from build123d import *

# Parameters (mm, degrees)
PAD_DEPTH       = 3.95
SKETCH001_W     = 110
SKETCH001_H     = 39.3
PAD001_DEPTH    = 50
SKETCH002_W     = 34.4
SKETCH002_H     = 46
POCKET_DEPTH    = 107
SKETCH003_W     = 46.5
SKETCH003_H     = 35
POCKET001_DEPTH = 40
CHAMFER_SIZE    = 2.5
CHAMFER001_SIZE = 5
FILLET_R        = 2.5
FILLET001_R     = 1
FILLET002_R     = 5
FILLET003_R     = 1


with BuildPart() as part:
    # Sketch → Pad (new body)
    with BuildSketch(Plane.XY):
        Polygon((7.25, 19.75), (45, 19.75), (45, -19.75), (24.75, -19.75), (24.75, -45.2), (63.35, -45.2), (63.35, -109.5), (-46.65, -109.5), (-46.65, -70.2), (-6.65, -70.2), (-6.65, -45.2), (7.25, -45.2), align=None)
    extrude(amount=PAD_DEPTH)

    # Sketch001 (on Face14 of Pad) → Pad001 (join)
    with BuildSketch(Plane.XY.offset(3.95)):
        with Locations((8.35, -89.85)):
            Rectangle(SKETCH001_W, SKETCH001_H)
    extrude(amount=PAD001_DEPTH)

    # Sketch002 (on Face15 of Pad001) → Pocket (cut)
    with BuildSketch(Plane.YZ.offset(63.35)):
        with Locations((-89.8, 28)):
            Rectangle(SKETCH002_W, SKETCH002_H)
    extrude(amount=-POCKET_DEPTH, mode=Mode.SUBTRACT)

    # Sketch003 (on Face1 of Pocket) → Pocket001 (cut)
    with BuildSketch(Plane.XY.offset(53.95)):
        with Locations((-17.9, -87.7)):
            Rectangle(SKETCH003_W, SKETCH003_H)
        with Locations((33.6, -87.7)):
            Rectangle(SKETCH003_W, SKETCH003_H)
    extrude(amount=-POCKET001_DEPTH, mode=Mode.SUBTRACT)

    # Chamfer
    chamfer_edges = [part.edges().sort_by_distance(p)[0] for p in [
        (7.25, 19.75, 1.975),
    ]]
    chamfer(chamfer_edges, length=CHAMFER_SIZE)

    # Chamfer001
    chamfer001_edges = [part.edges().sort_by_distance(p)[0] for p in [
        (63.35, -45.2, 1.975),
    ]]
    chamfer(chamfer001_edges, length=CHAMFER001_SIZE)

    # Fillet
    fillet_edges = [part.edges().sort_by_distance(p)[0] for p in [
        (-6.65, -45.2, 1.975),
        (-6.65, -70.2, 1.975),
    ]]
    fillet(fillet_edges, radius=FILLET_R)

    # Fillet001
    fillet001_edges = [part.edges().sort_by_distance(p)[0] for p in [
        (9.85, -107, 51),
        (9.85, -107, 5),
        (9.85, -72.6, 5),
        (60.1, -72.6, 51),
        (7.85, -72.6, 51),
        (-42.4, -72.6, 51),
    ]]
    fillet(fillet001_edges, radius=FILLET001_R)

    # Fillet002
    fillet002_edges = [part.edges().sort_by_distance(p)[0] for p in [
        (-41.15, -105.2, 52.475),
        (5.35, -105.2, 52.475),
        (10.35, -105.2, 52.475),
        (56.85, -105.2, 52.475),
        (-41.15, -71.4, 13.95),
        (5.35, -71.4, 13.95),
        (10.35, -71.4, 13.95),
        (56.85, -71.4, 13.95),
        (-43.9, -70.2, 53.95),
        (7.85, -70.2, 53.95),
        (60.1, -70.2, 53.95),
    ]]
    fillet(fillet002_edges, radius=FILLET002_R)

    # Fillet003
    fillet003_edges = [part.edges().sort_by_distance(p)[0] for p in [
        (8.35, -109.5, 53.95),
        (-46.65, -109.5, 26.975),
        (63.35, -109.5, 26.975),
        (-46.65, -92.35, 53.95),
        (-46.65, -71.664466, 52.485534),
        (-46.65, -70.2, 24.475),
        (63.35, -70.2, 26.45),
        (63.35, -71.664466, 52.485534),
        (63.35, -92.35, 53.95),
        (8.35, -109.5, 0),
    ]]
    fillet(fillet003_edges, radius=FILLET003_R)


solid = part.part
Geometry check sheet. Reference: the model listing, model coordinates, mm. A direction names the side the tool comes from. Round coordinates to 2 decimals unless told otherwise and drop trailing zeros. Order: outer loops, then holes, each group sorted by start corner. A loop starts at its lowest first (then second) coordinate and runs counter-clockwise, first axis right, second up. Notation, with made-up numbers: M 52,-33 L 60,-33 A8 cw 60,-27 Z; hole C -8.5,61 d3. An arc over 180 degrees is marked long. Answer in a Markdown table with one row per item. Add a question column.
Item 1: Sectioned sample at D-D, the plane x = -12. Enter the section's corners in (y, z), plus the area to 3 significant figures.
Item 2: Sectioned sample at A-A, the plane y = -95.5. Enter the section's corners in (x, z), plus the area to 3 significant figures.
Item 3: Sectioned sample at C-C, the plane x = 28. Enter the section's corners in (y, z).
Item 4: Draft check along X on faces 5 (the face through (3.85, -103.77, 52.45)), 6 (the face through (20, -35, 3.95)), 7 (the face through (-6.65, -58, 2)). Enter one of: released by +X, released by -X, zero draft, split by the parting line, or undercut.
Item 5: Set-up check for faces 1 (the face through (35, -19.75, 2)), 2 (the face through (-41.15, -72, 44)), 3 (the face through (-43.65, -90, 28)), 4 (the face through (9, -58, 0)): record each of +Z, -Z, +X, -X, +Y, -Y from which the full face is reachable in a straight line by a thin tool's end or side.
Item 6: Depth check by flat-ended pin: pin 1 Ø1.2 at (y, z) = (-37.5, 2) entering from +X; pin 2 Ø4.5 at (x, z) = (3.5, 2.5) entering from +Y; pin 3 Ø3 at (y, z) = (-1, 2.5) entering from -X. Enter the tip coordinate at first touch or a pass-through.
Item 7: Material ranges on L1, parallel to Y at x = 47, z = 10; L2, parallel to Y at x = 32, z = 3; L3, parallel to Z at x = -41, y = -78, recorded low to high. Write a range as [from, to].
Item 8: Sectioned sample at B-B, the plane z = 21. Enter the section's corners in (x, y).
Filled in:
| question | item | result |
|---|---|---|
| 1 | outline | M -109.5,1 A1 ccw -108.5,0 L -70.2,0 L -70.2,13.95 L -72.6,13.95 L -72.6,6 A1 cw -73.6,5 L -106,5 A1 cw -107,6 L -107,50 A1 cw -106,51 L -105.2,51 L -105.2,53.95 L -108.5,53.95 A1 ccw -109.5,52.95 Z |
| 1 | area | 346 mm² |
| 2 | outline | M -46.65,0 L 63.35,0 L 63.35,5 L -43.65,5 L -43.65,51 L -41.15,51 L -41.15,53.95 L -45.65,53.95 A1 ccw -46.65,52.95 Z; M 5.35,51 L 10.35,51 L 10.35,53.95 L 5.35,53.95 Z; M 56.85,51 L 63.35,51 L 63.35,52.95 A1 ccw 62.35,53.95 L 56.85,53.95 Z |
| 2 | area | 738 mm² |
| 3 | outline | M -109.5,1 A1 ccw -108.5,0 L -45.2,0 L -45.2,3.95 L -70.2,3.95 L -70.2,13.95 L -72.6,13.95 L -72.6,6 A1 cw -73.6,5 L -106,5 A1 cw -107,6 L -107,50 A1 cw -106,51 L -105.2,51 L -105.2,53.95 L -108.5,53.95 A1 ccw -109.5,52.95 Z; M -19.75,0 L 19.75,0 L 19.75,3.95 L -19.75,3.95 Z |
| 4 | face 5 | undercut |
| 4 | face 6 | zero draft |
| 4 | face 7 | released by -X |
| 5 | face 1 | +Z, -Z, +X |
| 5 | face 2 | +Z, +Y |
| 5 | face 3 | +X |
| 5 | face 4 | -Z, +X, -X, +Y, -Y |
| 6 | pin 1 | stops at x = 24.75 |
| 6 | pin 2 | stops at y = -45.2 |
| 6 | pin 3 | stops at x = 7.25 |
| 7 | L1 | y = [-109.5, -107], [-72.6, -70.2] |
| 7 | L2 | y = [-109.5, -45.2], [-19.75, 19.75] |
| 7 | L3 | z = [0, 5] |
| 8 | outline | M -46.65,-108.5 A1 ccw -45.65,-109.5 L 62.35,-109.5 A1 ccw 63.35,-108.5 L 63.35,-107 L -43.65,-107 L -43.65,-72.6 L -41.15,-72.6 L -41.15,-70.2 L -45.65,-70.2 A1 ccw -46.65,-71.2 Z; M 5.35,-72.6 L 10.35,-72.6 L 10.35,-70.2 L 5.35,-70.2 Z; M 56.85,-72.6 L 63.35,-72.6 L 63.35,-71.2 A1 ccw 62.35,-70.2 L 56.85,-70.2 Z |
